For this review, take the finished solid that the model builds, in its own axes (mm). A direction names the side the tool comes from. Round coordinates to 2 decimals unless told otherwise and drop trailing zeros. Write each loop counter-clockwise with the first axis right and the second up, starting at its lowest first coordinate (ties: lowest second). Pieces come first, ordered by that corner, then holes. Notation, with made-up numbers: M 75,74 L 122,74 A10 ccw 122,79 Z; hole C -27,-32 d4. An arc over 180 degrees is marked long. Write each question's results on one line, items separated by ' | '. Start each with the question number.
```python
from build123d import *

# Parameters (mm, degrees)
SKETCH_3_R                   = 48.25
SKETCH_3_R_2                 = 32.5
EXTRUDE_2_DEPTH              = 3
SKETCH_5_R                   = 41.525287223
SKETCH_5_R_2                 = 39.197474278
EXTRUDE_3_DEPTH              = 0.1
EXTRUDE_START                = -3
SKETCH_2_R                   = 48.25
SKETCH_2_R_2                 = 32.5
EXTRUDE_1_DEPTH              = 3
EXTRUDE_5_DEPTH              = 3
EXTRUDE_5_DEPTH_BACK         = 2.98
HOLE_WIZARD_M3_5_1_D         = 2.9
EXTRUDE_7_DEPTH              = 4
EXTRUDE_7_DEPTH_BACK         = 2
CUT_EXTRUDE_10_DEPTH         = 88.222318818
CUT_EXTRUDE_10_DEPTH_BACK    = 88.222318818
HOLE_WIZARD_M4_3_D           = 4.5
HOLE_WIZARD_M4_3_CBORE_D     = 8
HOLE_WIZARD_M4_3_CBORE_DEPTH = 4
FILLET_1_R                   = 2
CUT_EXTRUDE_11_DEPTH         = 10
CUT_EXTRUDE_11_DEPTH_BACK    = 10
FILLET_2_R                   = 3
SKETCH_33_R                  = 3.5
CUT_EXTRUDE_12_DEPTH         = 4
FILLET_5_R                   = 2


with BuildPart() as part:
    # 草图3 → 凸台-拉伸2 (new body)
    with BuildSketch(Plane.XY):
        Circle(SKETCH_3_R)
        Circle(SKETCH_3_R_2, mode=Mode.SUBTRACT)
    extrude(amount=EXTRUDE_2_DEPTH)

    # 草图5 → 凸台-拉伸3 (add)
    with BuildSketch(Plane.XY.offset(3)):
        Circle(SKETCH_5_R)
        Circle(SKETCH_5_R_2, mode=Mode.SUBTRACT)
    extrude(amount=-EXTRUDE_3_DEPTH)

    # 草图2 → 凸台-拉伸1 (add)
    with BuildSketch(Plane.XY.offset(EXTRUDE_START)):
        Circle(SKETCH_2_R)
        Circle(SKETCH_2_R_2, mode=Mode.SUBTRACT)
    extrude(amount=EXTRUDE_1_DEPTH)

    # 草图8 → 凸台-拉伸5 (add, two sides: drawn at the far end of the back side and taken through both)
    with BuildSketch(Plane.XY.offset(-EXTRUDE_5_DEPTH_BACK)):
        with BuildLine():
            Line((-57, 20.010872518), (-47.592541309, 20.010872518))
            ThreePointArc((-47.592541309, 20.010872518), (-44.543901449, 20.847255835), (-42.348850377, 23.12222679))
            ThreePointArc((-42.348850377, 23.12222679), (-48.25, 0), (-42.348850377, -23.12222679))
            ThreePointArc((-42.348850377, -23.12222679), (-44.543901449, -20.847255835), (-47.592541309, -20.010872518))
            Line((-47.592541309, -20.010872518), (-57, -20.010872518))
            Line((-57, -20.010872518), (-57, 20.010872518))
        make_face()
    extrude(amount=EXTRUDE_5_DEPTH + EXTRUDE_5_DEPTH_BACK)

    # M3.5 螺纹孔的螺纹孔钻头1 (through all)
    with Locations(Plane(origin=(31.466251763, 31.466251763, 3), x_dir=(1, 0, 0), z_dir=(0, 0, 1))):
        with Locations((0, 0), (13.033748237, -31.466251763), (0, -62.932503526), (-62.932503526, -62.932503526), (-75.966251763, -31.466251763), (-62.932503526, 0), (-31.466251763, -73.966251763), (-31.466251763, 11.033748237)):
            Hole(HOLE_WIZARD_M3_5_1_D / 2)

    # 草图26 → 凸台-拉伸7 (add, two sides: drawn at the far end of the back side and taken through both)
    with BuildSketch(Plane.ZY.offset(57).offset(-EXTRUDE_7_DEPTH_BACK)):
        with BuildLine():
            ThreePointArc((-12.98, 26.5), (-39.48, 0), (-12.98, -26.5))
            ThreePointArc((-12.98, -26.5), (-9.999377331, -25.617338519), (-7.98, -23.254010785))
            ThreePointArc((-7.98, -23.254010785), (-5.960622669, -20.89068305), (-2.98, -20.008021569))
            Line((-2.98, -20.008021569), (3, -20.008021569))
            Line((3, -20.008021569), (3, 20.010872518))
            Line((3, 20.010872518), (-2.98, 20.010872518))
            ThreePointArc((-2.98, 20.010872518), (-5.959846717, 20.892654018), (-7.98, 23.254010785))
            ThreePointArc((-7.98, 23.254010785), (-10.000085555, 25.616247597), (-12.98, 26.5))
        make_face()
    extrude(amount=EXTRUDE_7_DEPTH + EXTRUDE_7_DEPTH_BACK)

    # 草图27 → 切除-拉伸10 (cut, two sides: drawn at the far end of the back side and taken through both)
    with BuildSketch(Plane.XY.offset(-CUT_EXTRUDE_10_DEPTH_BACK)):
        with BuildLine():
            Line((10, -47.202356933), (10, 47.202356933))
            ThreePointArc((10, 47.202356933), (48.25, 0), (10, -47.202356933))
        make_face()
    extrude(amount=CUT_EXTRUDE_10_DEPTH + CUT_EXTRUDE_10_DEPTH_BACK, mode=Mode.SUBTRACT)

    # M4 六角凹头盖的柱孔3 (through all)
    with Locations(Plane(origin=(-55, 17.25, -12.98), x_dir=(0, 0, 1), z_dir=(1, 0, 0))):
        with Locations((0, 0), (-14.938938215, 8.625), (-14.938938215, 25.875), (0, 34.5)):
            CounterBoreHole(HOLE_WIZARD_M4_3_D / 2, HOLE_WIZARD_M4_3_CBORE_D / 2, HOLE_WIZARD_M4_3_CBORE_DEPTH)

    # 圆角1
    fillet_1_edges = [part.edges().sort_by_distance(p)[0] for p in [
        (-61, 0.001425474, 3),
    ]]
    fillet(fillet_1_edges, radius=FILLET_1_R)

    # 草图30 → 切除-拉伸11 (cut, two sides: drawn at the far end of the back side and taken through both)
    with BuildSketch(Plane.ZY.offset(57).offset(-CUT_EXTRUDE_11_DEPTH_BACK)):
        with BuildLine():
            Line((-12.98, 8.39165306), (-12.98, -8.39165306))
            ThreePointArc((-12.98, -8.39165306), (-21.37165306, 0), (-12.98, 8.39165306))
        make_face()
    extrude(amount=CUT_EXTRUDE_11_DEPTH + CUT_EXTRUDE_11_DEPTH_BACK, mode=Mode.SUBTRACT)

    # 圆角2
    fillet_2_edges = [part.edges().sort_by_distance(p)[0] for p in [
        (-58, -8.39165306, -12.98),
        (-58, 8.39165306, -12.98),
    ]]
    fillet(fillet_2_edges, radius=FILLET_2_R)

    # 草图33 → 切除-拉伸12 (cut)
    with BuildSketch(Plane.XY.offset(3)):
        with Locations((0, 42.5)):
            Circle(SKETCH_33_R)
        with Locations((0, -42.5)):
            Circle(SKETCH_33_R)
        with Locations((-31.466251763, 31.466251763)):
            Circle(SKETCH_33_R)
        with Locations((-44.5, 0)):
            Circle(SKETCH_33_R)
        with Locations((-31.466251763, -31.466251763)):
            Circle(SKETCH_33_R)
    extrude(amount=-CUT_EXTRUDE_12_DEPTH, mode=Mode.SUBTRACT)

    # 圆角5
    # the kernel refuses this fillet: 2 mm, written as the material it adds along each edge
    with BuildSketch(Plane(origin=(-55, -25.008021569, -2.98), x_dir=(0, 0, -1), z_dir=(0, 1, 0))) as fillet_5_piece_1_section:
        with BuildLine():
            CenterArc((FILLET_5_R, -FILLET_5_R), FILLET_5_R, 90, 90)
            Line((0, -FILLET_5_R), (0, 0))
            Line((0, 0), (FILLET_5_R, 0))
        make_face()
    fillet_5_piece_1 = extrude(amount=50.018894088, mode=Mode.PRIVATE)
    fillet_5_piece_1 = fillet_5_piece_1 - Plane(origin=(-54.891551476, 25.486733073, -2.98), x_dir=(0, -1, 0), z_dir=(1, 0, 0)) * Cylinder(5.475860555, 109, mode=Mode.PRIVATE)
    fillet_5_piece_1 = fillet_5_piece_1 - Plane(origin=(-54.891551476, -25.481922379, -2.98), x_dir=(0, 0.40700620484751754, -0.9134253933494627), z_dir=(1, 0, 0)) * Cylinder(5.473900809, 109, mode=Mode.PRIVATE)
    add(fillet_5_piece_1)


solid = part.part
```
Item 1: Mouldability with a two-part tool opening along Y and no side actions: class faces 6 (the cylindrical face through (-54.43, -0.28, -3.58)), 7 (the cylindrical face through (-56.972, 13.877, -10.83)), 8 (the flat face through (-54, 20.011, 0)) as pulls with the +Y half, pulls with the -Y half, needs draft (parallel to the pull), parting line crosses it, or undercut.
Item 2: We need section D-D on x = -16. State the section outline as (y, z) points, then the cut area to 3 significant figures.
Item 3: For probe 1 along Y at (x, z) = (0, -2.2); probe 2 along Z at (x, y) = (-17.5, -34); probe 3 along X at (y, z) = (-7.5, -11.5), list the stretches that pass through material, from the lowest coordinate up.
Item 4: For faces 1 (the cylindrical face through (-43.05, 0.06, -2.01)), 2 (the cylindrical face through (0, -39, 1)), 3 (the cylindrical face through (-60.43, 0.28, 2.4)), 4 (the cylindrical face through (-58.042, 7.105, -14.527)), 5 (the cylindrical face through (-56.972, -7.093, -24.224)), list the 3-axis set-ups (+Z, -Z, +X, -X, +Y, -Y) from which the entire face can be reached by the end or side of a thin tool; tool diameter is ignored.
Item 5: We need section A-A on x = 0. State the section outline as (y, z) points, then the cut area to 3 significant figures.
Item 6: We need section C-C on z = -27. State the section outline as (x, y) points.
Item 7: Insertion check: P1, Ø13, axis at y = 8.62, z = -27.92, coming from the +X side; P2, Ø2, axis at x = 1, y = 42.5, coming from the +Z side; P3, Ø1.7, axis at x = -31.47, y = 31.47, coming from the +Z side; P4, Ø3, axis at x = -57, z = -0.5, coming from the +Y side. Each pin has a flat end and moves straight along its axis. Give the tip position at first contact, or say it passes through.
Numbers:
1) face 6: needs draft | face 7: undercut | face 8: pulls with the +Y half
2) outline: M -45.52,-3 L -28.29,-3 L -28.29,3 L -45.52,3 Z; M 28.29,-3 L 45.52,-3 L 45.52,3 L 28.29,3 Z | area: 207 mm^2
3) probe 1: y = -48.25 to -43.95, -41.05 to -32.5, 32.5 to 41.05, 43.95 to 48.25 | probe 2: z = -3 to 3 | probe 3: x = -61 to -55
4) face 1: +Z, -Z | face 2: +Z | face 3: +Z, -X, +Y, -Y | face 4: +X, -X | face 5: +X
5) outline: M -48.25,-3 L -43.95,-3 L -43.95,-1 L -46,-1 L -46,3 L -48.25,3 Z; M -41.05,-3 L -32.5,-3 L -32.5,3 L -39,3 L -39,-1 L -41.05,-1 Z; M 32.5,-3 L 41.05,-3 L 41.05,-1 L 39,-1 L 39,3 L 32.5,3 Z; M 43.95,-3 L 48.25,-3 L 48.25,3 L 46,3 L 46,-1 L 43.95,-1 Z | area: 121 mm^2
6) outline: M -61,-22.49 L -55,-22.49 L -55,-12.52 L -59,-12.52 L -59,-10.68 L -61,-10.68 Z; M -61,-6.57 L -59,-6.57 L -59,-4.73 L -55,-4.73 L -55,4.73 L -59,4.73 L -59,6.57 L -61,6.57 Z; M -61,10.68 L -59,10.68 L -59,12.52 L -55,12.52 L -55,22.49 L -61,22.49 Z
7) P1: stops at x = -55 | P2: stops at z = -1 | P3: passes through | P4: stops at y = 20.01
